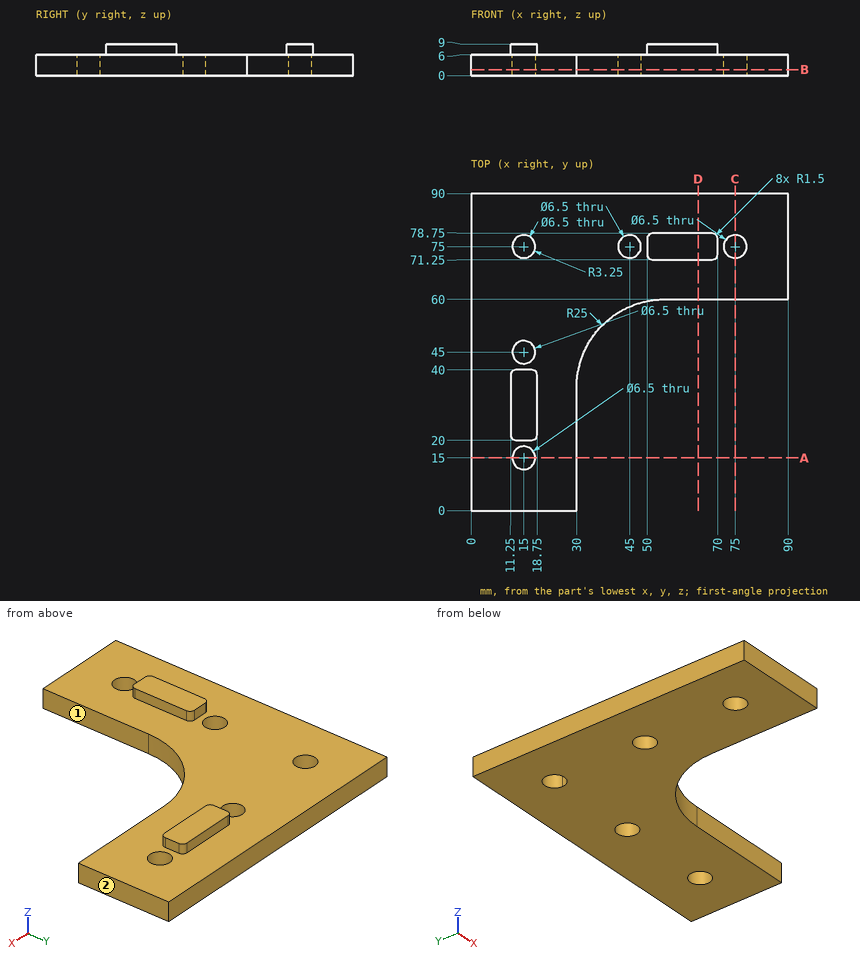
Verification items for this drawing (mm, ordinates from the low corner). A direction names the side the tool comes from. Round coordinates to 2 decimals unless told otherwise and drop trailing zeros. Loops run counter-clockwise (first coordinate to the right, second up) from the corner with the lowest first, then second, coordinate; pieces in that order, holes last. Notation, with made-up numbers: M -2,4.5 L 20,4.5 A27 cw 20,33.5 Z; hole C 71,75.5 d5. An arc over 180 degrees is marked long. Answer as a JSON object with one key per item and string values.
1. Scan lines: line 1 (Y direction, x = 15, z = 3.9); line 2 (Z direction, x = 63, y = 80); line 3 (Y direction, x = 85.5, z = 4.5). Record each from-to range of solid material in increasing order.
Reply:
{"line 1": "y = 0 to 11.75, 18.25 to 41.75, 48.25 to 71.75, 78.25 to 90", "line 2": "z = 0 to 6", "line 3": "y = 60 to 90"}
2. Gauge pin test, flat ends, axial feed: P1, Ø5, axis at x = 15, y = 45, coming from the -Z side; P2, Ø2.5, axis at x = 63, z = 8, coming from the +Y side; P3, Ø1.5, axis at x = 14, z = 8, coming from the -Y side; P4, Ø3, axis at y = 11.5, z = 2.5, coming from the +X side. Record the tip position at first contact, or that the pin passes through.
Reply:
{"P1": "passes through", "P2": "stops at y = 78.75", "P3": "stops at y = 20", "P4": "stops at x = 30"}
3. Section check A-A (y = 15). Record the boundary of the cut face in (x, z).
Reply:
{"outline": "M 0,0 L 11.75,0 L 11.75,6 L 0,6 Z; M 18.25,0 L 30,0 L 30,6 L 18.25,6 Z"}
4. Access from +Z, -Z, +X, -X, +Y, -Y to the whole of each face (thin tool, end or side, straight path). Record for the marked faces 1 and 2.
Reply:
{"face 1": "+Z, -Z, +X, -Y", "face 2": "+Z, -Z, +X, +Y, -Y"}
5. Section check C-C (x = 75). Record the boundary of the cut face in (y, z), plus the area to 3 significant figures.
Reply:
{"outline": "M 60,0 L 71.75,0 L 71.75,6 L 60,6 Z; M 78.25,0 L 90,0 L 90,6 L 78.25,6 Z", "area": "141 mm²"}
6. Section check D-D (x = 64.5). Record the boundary of the cut face in (y, z), plus the area to 4 significant figures.
Reply:
{"outline": "M 60,0 L 90,0 L 90,6 L 78.75,6 L 78.75,9 L 71.25,9 L 71.25,6 L 60,6 Z", "area": "202.5 mm²"}
7. Section check B-B (z = 1.75). Record the boundary of the cut face in (x, y).
Reply:
{"outline": "M 0,0 L 30,0 L 30,35 A25 cw 55,60 L 90,60 L 90,90 L 0,90 Z; hole C 15,15 d6.5; hole C 15,45 d6.5; hole C 15,75 d6.5; hole C 45,75 d6.5; hole C 75,75 d6.5"}
